from build123d import *

# Parameters (mm, degrees)
SKETCH20_W            = 129.286
SKETCH20_H            = 70.104
BOSS_EXTRUDE5_DEPTH   = 1.699999902
BOSS_EXTRUDE6_DEPTH   = 1.7
FILLET3_R             = 2.54
F_4_40_TAPPED_HOLE3_D = 2.2606
SKETCH28_W            = 12.7
SKETCH28_H            = 10.16
SKETCH28_W_2          = 15.24
SKETCH28_H_2          = 8.382
SKETCH28_W_3          = 12.446
SKETCH28_H_3          = 5.842
CUT_EXTRUDE1_DEPTH    = 2.54


with BuildPart() as part:
    # Sketch20 → Boss-Extrude5 (new body)
    with BuildSketch(Plane(origin=(0, 0, 0), x_dir=(1, 0, 0), z_dir=(0, 1, 0))):
        with Locations((62.643, 54.832)):
            Rectangle(SKETCH20_W, SKETCH20_H)
    extrude(amount=-BOSS_EXTRUDE5_DEPTH)

    # Sketch20_3 → Boss-Extrude6 (add)
    with BuildSketch(Plane(origin=(0, 0, 0), x_dir=(1, 0, 0), z_dir=(0, 1, 0))):
        with BuildLine():
            Line((2.572, 21.812), (122.714, 21.812))
            ThreePointArc((122.714, 21.812), (123.457948776, 23.608051224), (125.254, 24.352))
            Line((125.254, 24.352), (125.254, 85.312))
            ThreePointArc((125.254, 85.312), (123.457948776, 86.055948776), (122.714, 87.852))
            Line((122.714, 87.852), (2.572, 87.852))
            ThreePointArc((2.572, 87.852), (1.828051224, 86.055948776), (0.032, 85.312))
            Line((0.032, 85.312), (0.032, 24.352))
            ThreePointArc((0.032, 24.352), (1.828051224, 23.608051224), (2.572, 21.812))
        make_face()
        with BuildLine():
            Line((3.624102448, 23.082), (121.661897552, 23.082))
            ThreePointArc((121.661897552, 23.082), (122.559923164, 24.506076836), (123.984, 25.404102448))
            Line((123.984, 25.404102448), (123.984, 84.259897552))
            ThreePointArc((123.984, 84.259897552), (122.559923164, 85.157923164), (121.661897552, 86.582))
            Line((121.661897552, 86.582), (3.624102448, 86.582))
            ThreePointArc((3.624102448, 86.582), (2.726076836, 85.157923164), (1.302, 84.259897552))
            Line((1.302, 84.259897552), (1.302, 25.404102448))
            ThreePointArc((1.302, 25.404102448), (2.726076836, 24.506076836), (3.624102448, 23.082))
        make_face(mode=Mode.SUBTRACT)
    extrude(amount=BOSS_EXTRUDE6_DEPTH)

    # Fillet3
    fillet3_edges = [part.edges().sort_by_distance(p)[0] for p in [
        (-2, -0.849999951, -89.884),
        (-2, -0.849999951, -19.78),
        (127.286, -0.849999951, -19.78),
        (127.286, -0.849999951, -89.884),
    ]]
    fillet(fillet3_edges, radius=FILLET3_R)

    # 4-40 Tapped Hole3 (through all)
    with Locations(Plane(origin=(0, 0, 0), x_dir=(1, 0, 0), z_dir=(0, 1, 0))):
        with Locations((0.032, 21.812), (125.254, 21.812), (125.254, 87.852), (0.032, 87.852)):
            Hole(F_4_40_TAPPED_HOLE3_D / 2)

    # Sketch28 → Cut-Extrude1 (cut)
    with BuildSketch(Plane.XZ.offset(1.699999902)):
        with Locations((27.337, -73.882)):
            Rectangle(SKETCH28_W, SKETCH28_H)
        with Locations((76.994, -59.404)):
            Rectangle(SKETCH28_W_2, SKETCH28_H_2)
        with Locations((27.21, -55.213)):
            Rectangle(SKETCH28_W_3, SKETCH28_H_3)
    extrude(amount=-CUT_EXTRUDE1_DEPTH, mode=Mode.SUBTRACT)


solid = part.part
The listing builds one solid part. Answer for the finished solid, in the listing's coordinates (mm). A direction names the side the tool comes from. Give positions to 0.01 mm unless a question says otherwise; leave off trailing zeros. Write each loop counter-clockwise with the first axis right and the second up, starting at its lowest first coordinate (ties: lowest second). Pieces come first, ordered by that corner, then holes. Notation, with made-up numbers: (17, 31.25) - (56, 31.25) arc R17 cw to (56, 64.25) - close; hole circle Ø6 at (66, 86). An arc over 180 degrees is marked (long way). One line per question, with ' | ' between items. Start each with the question number.
1. Section A-A, the plane x = 25 is taken. Determine the outline of the cut face in (y, z), then the cut area to 3 significant figures.
2. Given P1, Ø0.8, axis at y = 1, z = -64, coming from the +X side; P2, Ø2.5, axis at x = 125.254, z = -21.812, coming from the +Y side; P3, Ø0.8, axis at y = 1, z = -54.5, coming from the -X side, each flat-ended and moving along its own axis, determine where each tip first touches the part or whether it passes through.
3. Section C-C, the plane y = 0.55 is taken. Determine the outline of the cut face in (x, z).
4. Straight lines are drawn through the part: line 1 (Z direction, x = 69, y = 0.5); line 2 (X direction, y = -1.6, z = -75.5); line 3 (X direction, y = 0.5, z = -60). For each, find the intervals that lie inside material, in ascending order.
5. Section D-D, the plane z = -67.5 is taken. Determine the outline of the cut face in (x, y), then the cut area to 3 significant figures.
6. Determine the mould class of faces 4 (the face through (62, 0, -89)), 5 (the face through (2.71, 0.84, -24.52)), 6 (the face through (0.28, -0.86, -86.75)), 7 (the face through (126.52, -0.86, -20.5)) for opening direction X: +X half, -X half, draft (parallel to the pull), parting line (faces both ways), or undercut.
7. Section B-B, the plane z = -54 is taken. Determine the outline of the cut face in (x, y), then the cut area to 3 significant figures.
8. For faces 1 (the face through (1.808, 0.838, -23.628)), 2 (the face through (1.85, 0.84, -86.08)), 3 (the face through (123.478, 0.838, -86.036)), determine the directions among +Z, -Z, +X, -X, +Y, -Y from which every point of the face is accessible in a straight line to the end or side of a thin tool.
Result:
1) outline: (-1.7, -89.88) - (0, -89.88) - (0, -87.85) - (1.7, -87.85) - (1.7, -86.58) - (0, -86.58) - (0, -78.96) - (-1.7, -78.96) - close; (-1.7, -68.8) - (0, -68.8) - (0, -58.13) - (-1.7, -58.13) - close; (-1.7, -52.29) - (0, -52.29) - (0, -23.08) - (1.7, -23.08) - (1.7, -21.81) - (0, -21.81) - (0, -19.78) - (-1.7, -19.78) - close | area: 96.3 mm2
2) P1: stops at x = 125.25 | P2: stops at y = 0 | P3: stops at x = 0.03
3) outline: (0.03, -85.31) arc R2.54 cw to (2.57, -87.85) - (122.71, -87.85) arc R2.54 cw to (125.25, -85.31) - (125.25, -24.35) arc R2.54 cw to (122.71, -21.81) - (2.57, -21.81) arc R2.54 cw to (0.03, -24.35) - close; hole (1.3, -84.26) arc R3.81 cw to (3.62, -86.58) - (121.66, -86.58) arc R3.81 cw to (123.98, -84.26) - (123.98, -25.4) arc R3.81 cw to (121.66, -23.08) - (3.62, -23.08) arc R3.81 cw to (1.3, -25.4) - close
4) line 1: z = -87.85 to -86.58, -23.08 to -21.81 | line 2: x = -2 to 20.99, 33.69 to 127.29 | line 3: x = 0.03 to 1.3, 123.98 to 125.25
5) outline: (-2, -1.7) - (127.29, -1.7) - (127.29, 0) - (125.25, 0) - (125.25, 1.7) - (123.98, 1.7) - (123.98, 0) - (1.3, 0) - (1.3, 1.7) - (0.03, 1.7) - (0.03, 0) - (-2, 0) - close | area: 224 mm2
6) face 4: draft | face 5: undercut | face 6: undercut | face 7: +X half
7) outline: (-2, -1.7) - (20.99, -1.7) - (20.99, 0) - (1.3, 0) - (1.3, 1.7) - (0.03, 1.7) - (0.03, 0) - (-2, 0) - close; (33.43, -1.7) - (127.29, -1.7) - (127.29, 0) - (125.25, 0) - (125.25, 1.7) - (123.98, 1.7) - (123.98, 0) - (33.43, 0) - close | area: 203 mm2
8) face 1: +Z, -X, +Y | face 2: -Z, -X, +Y | face 3: -Z, +X, +Y
